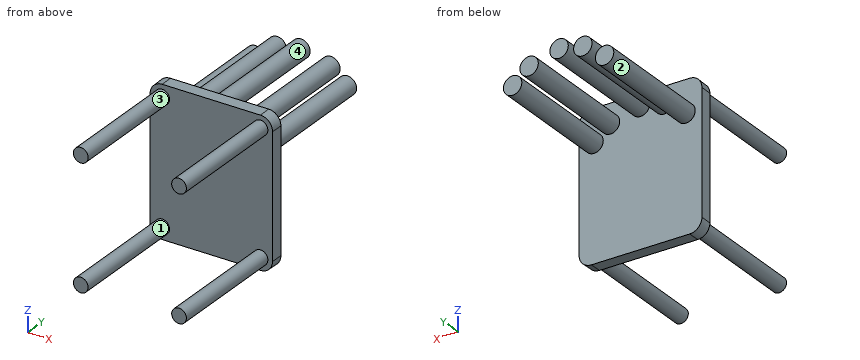
from build123d import *

# Parameters (mm, degrees)
F1_DEPTH = 10
F1_TAPER = 1
F2_R     = 6
F3_DEPTH = 100
F4_R     = 7.5
F5_DEPTH = 100


with BuildPart() as f1:
    # F0 (on Front) → F1 (new body)
    with BuildSketch(Plane.XZ):
        with BuildLine():
            ThreePointArc((50, 50), (47.0710678119, 57.0710678119), (40, 60))
            Line((40, 60), (-40, 60))
            ThreePointArc((-40, 60), (-47.0710678119, 57.0710678119), (-50, 50))
            Line((-50, 50), (-50, -50))
            ThreePointArc((-50, -50), (-47.0710678119, -57.0710678119), (-40, -60))
            Line((-40, -60), (40, -60))
            ThreePointArc((40, -60), (47.0710678119, -57.0710678119), (50, -50))
            Line((50, -50), (50, 50))
        make_face()
    extrude(amount=F1_DEPTH, taper=F1_TAPER)

    # F2 (on face) → F3 (join)
    with BuildSketch(Plane.XZ.offset(10)):
        with Locations((-40, 50)):
            Circle(F2_R)
        with Locations((40, 50)):
            Circle(F2_R)
        with Locations((40, -50)):
            Circle(F2_R)
        with Locations((-40, -50)):
            Circle(F2_R)
    extrude(amount=F3_DEPTH)

    # F4 (on face) → F5 (join)
    with BuildSketch(Plane(origin=(0, 0, 0), x_dir=(-1, 0, 0), z_dir=(0, 1, 0))):
        with Locations((-37.8239102132, 32.7009451879)):
            Circle(F4_R)
        with Locations((-24.4146151623, 43.6340069955)):
            Circle(F4_R)
        with Locations((1.0837e-06, 49.8871542513)):
            Circle(F4_R)
        with Locations((19.318186678, 46.0232570767)):
            Circle(F4_R)
        with Locations((37.0454452932, 33.7496697903)):
            Circle(F4_R)
    extrude(amount=F5_DEPTH)


solid = f1.part
Read the model definition and answer for the solid it produces. Units are mm, in the model's axes. Face numbers are marked on the shaded views. A direction names the side the tool comes from. Give positions to 0.01 mm unless a question says otherwise; leave off trailing zeros. Loops run counter-clockwise (first coordinate to the right, second up) from the corner with the lowest first, then second, coordinate; pieces in that order, holes last. Notation, with made-up numbers: (15, -2.5) -> (32, -2.5) arc R10 ccw to (32, 4.5) -> close; hole circle Ø2 at (42, -7). An arc over 180 degrees is marked (long way). Use a Markdown table: item, result.
Q1. Each of these flat-tipped pins is pushed along its axis until it touches: pin 1 (3 mm diameter, centred on x = 34.5, z = 12.5, fed in from +Y); pin 2 (10 mm diameter, centred on x = 13.5, z = -5, fed in from -Y); pin 3 (3 mm diameter, centred on x = 7.5, y = 35.5, fed in from -Z). Where does it stop, or does it pass through?
Solved:
| item | result |
|---|---|
| pin 1 | stops at y = 0 |
| pin 2 | stops at y = -10 |
| pin 3 | stops at z = 45.39 |
Q2. Find the intervals of material crossed by line 1 along Z through (x, y) = (39.5, -61); line 2 along Y through (x, z) = (-23, -22.5); line 3 along Y through (x, z) = (-25, 42.5), in increasing order.
Solved:
| item | result |
|---|---|
| line 1 | z = -55.98 to -44.02, 44.02 to 55.98 |
| line 2 | y = -10 to 0 |
| line 3 | y = -10 to 100 |
Q3. Section B-B, the plane y = 40.5 is taken. Determine the outline of the cut face in (x, z), then the cut area to 3 significant figures.
Solved:
| item | result |
|---|---|
| outline | circle Ø15 at (-37.05, 33.75); circle Ø15 at (-19.32, 46.02); circle Ø15 at (0, 49.89); circle Ø15 at (24.41, 43.63); circle Ø15 at (37.82, 32.7) |
| area | 884 mm^2 |
Q4. Determine the mould class of the marked faces 1 and 2 for opening direction Z: pulls with the +Z half, pulls with the -Z half, needs draft (parallel to the pull), parting line crosses it, or undercut.
Solved:
| item | result |
|---|---|
| face 1 | undercut |
| face 2 | parting line crosses it |
Q5. A tool of negligible diameter and unlimited length cuts with its end or side. For the marked faces 3 and 4, from which of +Z, -Z, +X, -X, +Y, -Y can it reach the whole face along a straight path? Write none if from no direction.
Solved:
| item | result |
|---|---|
| face 3 | -Y |
| face 4 | +Y |
Q6. Section A-A, the plane y = -48 is taken. Determine the outline of the cut face in (x, z).
Solved:
| item | result |
|---|---|
| outline | circle Ø12 at (-40, -50); circle Ø12 at (-40, 50); circle Ø12 at (40, -50); circle Ø12 at (40, 50) |
